Read the model definition and answer for the solid it produces. Units are mm, in the model's axes. A direction names the side the tool comes from. Round coordinates to 2 decimals unless told otherwise and drop trailing zeros. Write each loop counter-clockwise with the first axis right and the second up, starting at its lowest first coordinate (ties: lowest second). Pieces come first, ordered by that corner, then holes. Notation, with made-up numbers: (-10, 40) -> (34, 40) arc R15 cw to (34, 60) -> close; hole circle Ø5 at (33, -26). An arc over 180 degrees is marked (long way). Return JSON: item names as keys, results as strings. Group by question number.
(1) A cutting plane is placed at D-D on z = 0.7. Give the vertices of the cut face in (x, y).
(2) Given pin 1 (1.5 mm diameter, centred on y = -1.5, z = 3.5, fed in from +X); pin 2 (3.5 mm diameter, centred on x = 8, y = 0, fed in from +Z); pin 3 (1 mm diameter, centred on x = -8.5, z = 2.5, fed in from -Y), each flat-ended and moving along its own axis, determine where each tip first touches the part or whether it passes through.
(3) A cutting plane is placed at A-A on z = 3.85. Give the vertices of the cut face in (x, y).
(4) For faces 4 (the cylindrical face through (1.17, 9.83, 3.73)), 5 (the cylindrical face through (-5.126, 5.586, 1.205)), determine the directions among +Z, -Z, +X, -X, +Y, -Y from which every point of the face is accessible in a straight line to the end or side of a thin tool.
(5) A cutting plane is placed at B-B on y = 0. Give the vertices of the cut face in (x, z).
(6) The mould has two halves that part along Y. Classify faces 1 (the flat face through (4, -2, 5.5)), 2 (the cylindrical face through (4.8, -5.78, 1.34)), 3 (the cylindrical face through (5.076, -9.759, 2.085)): released by +Y, released by -Y, zero draft, split by the parting line, or undercut.
(7) Straight lines are drawn through the part: line 1 (Y direction, x = 0, z = 3.4); line 2 (Y direction, x = -0.25, z = 5); line 3 (Z direction, x = 4.5, y = -6). For each, find the intervals that lie inside material, in ascending order.
```python
from build123d import *

# Parameters (mm, degrees)
SKETCH2_R           = 11
SKETCH2_R_2         = 4.318
SKETCH2_R_3         = 1
BOSS_EXTRUDE1_DEPTH = 2
SKETCH3_R           = 11
SKETCH3_R_2         = 4.318
SKETCH3_R_3         = 2.171511002
BOSS_EXTRUDE2_DEPTH = 3.5
SKETCH5_R           = 1.5
CUT_EXTRUDE1_DEPTH  = 127
FILLET1_R           = 1.27


with BuildPart() as part:
    # Sketch2 → Boss-Extrude1 (new body)
    with BuildSketch(Plane.XY):
        Circle(SKETCH2_R)
        Circle(SKETCH2_R_2, mode=Mode.SUBTRACT)
        with Locations((0, 8)):
            Circle(SKETCH2_R_3, mode=Mode.SUBTRACT)
        with Locations((8, 0)):
            Circle(SKETCH2_R_3, mode=Mode.SUBTRACT)
        with Locations((0, -8)):
            Circle(SKETCH2_R_3, mode=Mode.SUBTRACT)
        with Locations((-8, 0)):
            Circle(SKETCH2_R_3, mode=Mode.SUBTRACT)
    extrude(amount=BOSS_EXTRUDE1_DEPTH)

    # Sketch3 → Boss-Extrude2 (add)
    with BuildSketch(Plane.XY.offset(2)):
        Circle(SKETCH3_R)
        Circle(SKETCH3_R_2, mode=Mode.SUBTRACT)
        with Locations((0, 8)):
            Circle(SKETCH3_R_3, mode=Mode.SUBTRACT)
        with Locations((8, 0)):
            Circle(SKETCH3_R_3, mode=Mode.SUBTRACT)
        with Locations((0, -8)):
            Circle(SKETCH3_R_3, mode=Mode.SUBTRACT)
        with Locations((-8, 0)):
            Circle(SKETCH3_R_3, mode=Mode.SUBTRACT)
    extrude(amount=BOSS_EXTRUDE2_DEPTH)

    # Sketch5 → Cut-Extrude1 (cut, symmetric)
    with BuildSketch(Plane(origin=(0, 0, 0), x_dir=(0.7071067811865477, 0.7071067811865475, 0), z_dir=(-0.7071067811865475, 0.7071067811865477, 0))):
        with Locations(Location((0, -2.668898501, 0), (0, 0, 180))):
            Circle(SKETCH5_R)
    extrude(amount=CUT_EXTRUDE1_DEPTH, both=True, mode=Mode.SUBTRACT)

    # Fillet1
    # the kernel refuses this fillet: 1.27 mm, written as the material it takes off along each edge
    with BuildSketch(Plane(origin=(0, 0, 5.5), x_dir=(1, 0, 0), z_dir=(0, -1, 0))) as fillet1_piece_1:
        with BuildLine():
            CenterArc((11 - FILLET1_R, -FILLET1_R), FILLET1_R, 0, 90)
            Line((11 - FILLET1_R, 0), (11, 0))
            Line((11, 0), (11, -FILLET1_R))
        make_face()
    revolve(axis=Axis((0, 0, 5.5), (0, 0, 1)), mode=Mode.SUBTRACT)


solid = part.part
```
Checks:
{
 "1": {"outline": "circle Ø22 at (0, 0); hole circle Ø2 at (-8, 0); hole circle Ø8.64 at (0, 0); hole circle Ø2 at (0, -8); hole circle Ø2 at (0, 8); hole circle Ø2 at (8, 0)"},
 "2": {"pin 1": "stops at x = 10.97", "pin 2": "stops at z = 2", "pin 3": "stops at y = -7.55"},
 "3": {"outline": "(-8.4, 7.1) arc R11 ccw to (7.1, -8.4) -> (2.33, -3.64) arc R4.32 cw to (-3.64, 2.33) -> close; (-7.1, 8.4) -> (-2.33, 3.64) arc R4.32 cw to (3.64, -2.33) -> (8.4, -7.1) arc R11 ccw to start; hole circle Ø4.34 at (-8, 0); hole circle Ø4.34 at (0, -8); hole circle Ø4.34 at (0, 8); hole circle Ø4.34 at (8, 0)"},
 "4": {"face 4": "+Z", "face 5": "none"},
 "5": {"outline": "(-11, 0) -> (-9, 0) -> (-9, 2) -> (-10.17, 2) -> (-10.17, 5.42) arc R1.27 ccw to (-11, 4.23) -> close; (-7, 0) -> (-4.32, 0) -> (-4.32, 5.5) -> (-5.83, 5.5) -> (-5.83, 2) -> (-7, 2) -> close; (4.32, 0) -> (7, 0) -> (7, 2) -> (5.83, 2) -> (5.83, 5.5) -> (4.32, 5.5) -> close; (9, 0) -> (11, 0) -> (11, 4.23) arc R1.27 ccw to (10.17, 5.42) -> (10.17, 2) -> (9, 2) -> close"},
 "6": {"face 1": "zero draft", "face 2": "undercut", "face 3": "split by the parting line"},
 "7": {"line 1": "y = -11 to -10.17, -5.83 to -4.32, 4.32 to 5.83, 10.17 to 11", "line 2": "y = -10.74 to -10.16, -5.84 to -4.31, 4.31 to 5.84, 10.16 to 10.74", "line 3": "z = 0 to 1.61, 3.73 to 5.5"}
}
